The model under review builds one solid part; all positions refer to its coordinate system, in mm. Face numbers are marked on the shaded views. A direction names the side the tool comes from. Round coordinates to 2 decimals unless told otherwise and drop trailing zeros. Answer as a JSON object with one key per item and string values. Group by question number.
Item 1: Consider section C-C (x = -37.5). State how many separate pieces and enclosed holes the cut face has, and give its area (3 significant figures).
Item 2: Tool access review of the marked faces 1, 2 and 3: name each direction out of +Z, -Z, +X, -X, +Y, -Y from which nothing blocks a thin tool from reaching the whole face with its end or side.
Item 3: Insertion check: P1, Ø3.5, axis at x = 0, y = -65, coming from the +Z side; P2, Ø3, axis at y = -8.5, z = 2.5, coming from the -X side. Each pin has a flat end and moves straight along its axis. Give the tip position at first contact, or say it passes through.
Item 4: To check wall thickness, follow line 1 (Y direction, x = -37.5, z = 2.8); line 2 (Y direction, x = -37.5, z = 2.7); line 3 (X direction, y = 64.5, z = 3.9). State the ranges of each line that lie inside material, in increasing order.
```python
from build123d import *

# Parameters (mm, degrees)
F0_R     = 1.5
F0_R_2   = 3
F1_DEPTH = 5
F2_R     = 4.99999


# Not quite as in the source:
# - a fillet or chamfer is up to 0.001 mm smaller than in the source, because OpenCascade refuses the exact size


with BuildPart() as f1:
    # F0 (on Top) → F1 (new body)
    with BuildSketch(Plane.XY):
        with BuildLine():
            Line((17.5, -65), (17.5, 65))
            ThreePointArc((17.5, 65), (0, 82.5), (-17.5, 65))
            Line((-17.5, 65), (-17.5, 38.903882032))
            ThreePointArc((-17.5, 38.903882032), (-18.5589728099, 35.826820985), (-21.2873218748, 34.0531695313))
            Line((-21.2873218748, 34.0531695313), (-53.7126781252, 25.9468304687))
            ThreePointArc((-53.7126781252, 25.9468304687), (-56.4410271901, 24.173179015), (-57.5, 21.096117968))
            Line((-57.5, 21.096117968), (-57.5, -21.096117968))
            ThreePointArc((-57.5, -21.096117968), (-56.4410271901, -24.173179015), (-53.7126781252, -25.9468304687))
            Line((-53.7126781252, -25.9468304687), (-21.2873218748, -34.0531695313))
            ThreePointArc((-21.2873218748, -34.0531695313), (-18.5589728099, -35.826820985), (-17.5, -38.903882032))
            Line((-17.5, -38.903882032), (-17.5, -65))
            ThreePointArc((-17.5, -65), (0, -82.5), (17.5, -65))
        make_face()
        with Locations((-37.5, -17.5)):
            Circle(F0_R, mode=Mode.SUBTRACT)
        with Locations((0, -65)):
            Circle(F0_R_2, mode=Mode.SUBTRACT)
        with Locations((-37.5, 17.5)):
            Circle(F0_R, mode=Mode.SUBTRACT)
        with Locations((0, 65)):
            Circle(F0_R_2, mode=Mode.SUBTRACT)
    extrude(amount=F1_DEPTH)

    # F2 (radius 5 in the source; OpenCascade refuses exactly that, so slightly less here)
    f2_edges = [f1.edges().sort_by_distance(p)[0] for p in [
        (17.5, 0, 0),
    ]]
    fillet(f2_edges, radius=F2_R)


solid = f1.part
```
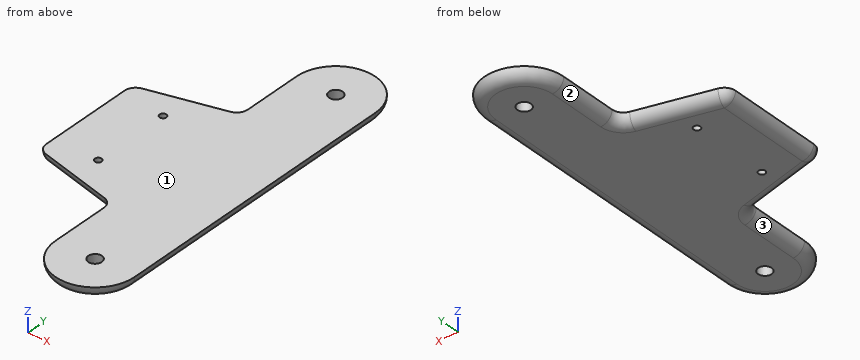
Geometry results:
{
 "1": {"separate pieces": "3", "enclosed holes": "0", "area": "259 mm^2"},
 "2": {"face 1": "+Z, +X, -X, +Y, -Y", "face 2": "-Z, -X, +Y", "face 3": "-Z, -X, -Y"},
 "3": {"P1": "passes through", "P2": "stops at x = -57.4"},
 "4": {"line 1": "y = -29.47 to -19, -16 to 16, 19 to 29.47", "line 2": "y = -29.42 to -19, -16 to 16, 19 to 29.42", "line 3": "x = -17.38 to -2.96, 2.96 to 17.38"}
}
